Here's how the part is built. I have some questions about the finished solid (model axes, mm). A direction names the side the tool comes from. Round coordinates to 2 decimals unless told otherwise and drop trailing zeros. Order: outer loops, then holes, each group sorted by start corner. A loop starts at its lowest first (then second) coordinate and runs counter-clockwise, first axis right, second up. Notation, with made-up numbers: (46, -19) - (57, -19) arc R9 cw to (57, -13) - close; hole circle Ø7 at (25.25, -4.5). An arc over 180 degrees is marked (long way). One line per item, written item: value.
from build123d import *

# Parameters (mm, degrees)
F1_W      = 22
F1_H      = 30
F2_DEPTH  = 8
F4_DEPTH  = 30.001
F6_DEPTH  = 2.5
F8_DEPTH  = 26
F9_W      = 3
F9_H      = 1.5
F10_DEPTH = 3


with BuildPart() as f2:
    # F1 (on Top) → F2 (new body)
    with BuildSketch(Plane.XY):
        with Locations((0, 15)):
            Rectangle(F1_W, F1_H)
    extrude(amount=-F2_DEPTH)

    # F3 (on face) → F4 (cut, through all)
    with BuildSketch(Plane.XZ):
        with BuildLine():
            Line((11, -8), (11, 0))
            ThreePointArc((11, 0), (10.100697, -4.356135), (7.549834, -8))
            Line((7.549834, -8), (11, -8))
        make_face()
        with BuildLine():
            ThreePointArc((-7.549834, -8), (-10.100697, -4.356135), (-11, 0))
            Line((-11, 0), (-11, -8))
            Line((-11, -8), (-7.549834, -8))
        make_face()
    extrude(amount=-F4_DEPTH, mode=Mode.SUBTRACT)

    # F5 (on face) → F6 (cut)
    with BuildSketch(Plane.XY):
        with BuildLine():
            ThreePointArc((-7.975, 5), (-9, 6.025), (-10.025, 5))
            Line((-10.025, 5), (-10.025, 3))
            ThreePointArc((-10.025, 3), (-9, 1.975), (-7.975, 3))
            Line((-7.975, 3), (-7.975, 5))
        make_face()
        with BuildLine():
            ThreePointArc((10.025, 5), (9, 6.025), (7.975, 5))
            Line((7.975, 5), (7.975, 3))
            ThreePointArc((7.975, 3), (9, 1.975), (10.025, 3))
            Line((10.025, 3), (10.025, 5))
        make_face()
        with BuildLine():
            ThreePointArc((-7.975, 27), (-9, 28.025), (-10.025, 27))
            Line((-10.025, 27), (-10.025, 25))
            ThreePointArc((-10.025, 25), (-9, 23.975), (-7.975, 25))
            Line((-7.975, 25), (-7.975, 27))
        make_face()
        with BuildLine():
            ThreePointArc((10.025, 27), (9, 28.025), (7.975, 27))
            Line((7.975, 27), (7.975, 25))
            ThreePointArc((7.975, 25), (9, 23.975), (10.025, 25))
            Line((10.025, 25), (10.025, 27))
        make_face()
    extrude(amount=-F6_DEPTH, mode=Mode.SUBTRACT)

    # F7 (on face) → F8 (cut)
    with BuildSketch(Plane.XZ):
        with BuildLine():
            Line((7, 0), (-7, 0))
            ThreePointArc((-7, 0), (-6.092572, -3.44682), (-3.605551, -6))
            Line((-3.605551, -6), (3.605551, -6))
            ThreePointArc((3.605551, -6), (6.092572, -3.44682), (7, 0))
        make_face()
    extrude(amount=-F8_DEPTH, mode=Mode.SUBTRACT)

    # F9 (on face) → F10 (cut)
    with BuildSketch(Plane.XZ.offset(-26)):
        with Locations((0, -0.75)):
            Rectangle(F9_W, F9_H)
    extrude(amount=-F10_DEPTH, mode=Mode.SUBTRACT)


solid = f2.part
Q1. If we section it at C-C, the plane x = 2.5: Please give me the cut outline in (y, z), then the cut area to 3 significant figures.
Results list:
outline: (0, -8) - (30, -8) - (30, 0) - (26, 0) - (26, -6) - (0, -6) - close
area: 84.0 mm²
Q2. If I drill on line 1 along Y through (x, z) = (-9, -0.25) (3 decimals); line 2 along Y through (x, z) = (-9.5, -1); line 3 along X through (y, z) = (5, -2.25) (3 decimals), over which ranges is the centre line in solid material (lowest first)?
Results list:
line 1: 0 to 1.975, 6.025 to 23.975, 28.025 to 30
line 2: 0 to 2.11, 5.89 to 24.11, 27.89 to 30
line 3: -10.767 to -10.025, -7.975 to -6.629, 6.629 to 7.975, 10.025 to 10.767
Q3. We'd pull the mould along X, two halves only. Please class faces 1 (the flat face through (-1.5, 27, -1)), 2 (the cylindrical face through (10.125, 14.79, -4.298)), 3 (the flat face through (0, 30, -4)): released by +X, released by -X, zero draft, split by the parting line, or undercut.
Results list:
face 1: undercut
face 2: released by +X
face 3: zero draft
Q4. If we section it at B-B, the plane z = -1: Please give me the cut outline in (x, y) (3 decimals), then the cut area to 3 significant figures.
Results list:
outline: (-10.954, 0) - (-6.928, 0) - (-6.928, 26) - (-1.5, 26) - (-1.5, 29) - (1.5, 29) - (1.5, 26) - (6.928, 26) - (6.928, 0) - (10.954, 0) - (10.954, 30) - (-10.954, 30) - close; hole (-10.025, 3) arc R1.025 ccw to (-7.975, 3) - (-7.975, 5) arc R1.025 ccw to (-10.025, 5) - close; hole (-10.025, 25) arc R1.025 ccw to (-7.975, 25) - (-7.975, 27) arc R1.025 ccw to (-10.025, 27) - close; hole (7.975, 3) arc R1.025 ccw to (10.025, 3) - (10.025, 5) arc R1.025 ccw to (7.975, 5) - close; hole (7.975, 25) arc R1.025 ccw to (10.025, 25) - (10.025, 27) arc R1.025 ccw to (7.975, 27) - close
area: 258 mm²
Q5. Will these pins go through, and if not, where does the flat tip stop? pin 1 (0.6 mm diameter, centred on y = 4, z = -1.5, fed in from -X); pin 2 (3 mm diameter, centred on y = 17.5, z = -5, fed in from +X); pin 3 (1.6 mm diameter, centred on y = 4, z = -1.5, fed in from +X); pin 4 (1.5 mm diameter, centred on x = -8, y = 15.5, fed in from -Z).
Results list:
pin 1: x = -10.93
pin 2: x = 10.43
pin 3: x = 10.98
pin 4: z = -8
Q6. Which directions (+Z, -Z, +X, -X, +Y, -Y) give clear straight access to the entire face, cutting with the end or side of a thin tool? Please do faces 4 (the cylindrical face through (-9.023, 23.975, -1.232)), 5 (the flat face through (0, 13, -6)), 6 (the flat face through (-7.5, 15.2, 0)).
Results list:
face 4: +Z
face 5: +Z, -Y
face 6: +Z, +X, -X, +Y, -Y
Q7. If we section it at D-D, the plane z = -4: Please give me the cut outline in (x, y), then the cut area to 3 significant figures.
Results list:
outline: (-10.25, 0) - (-5.74, 0) - (-5.74, 26) - (5.74, 26) - (5.74, 0) - (10.25, 0) - (10.25, 30) - (-10.25, 30) - close
area: 316 mm²
Q8. If we section it at A-A, the plane y = 13.25: Please give me the cut outline in (x, z).
Results list:
outline: (-11, 0) arc R11 ccw to (-7.55, -8) - (7.55, -8) arc R11 ccw to (11, 0) - (7, 0) arc R7 cw to (3.61, -6) - (-3.61, -6) arc R7 cw to (-7, 0) - close
